```python
from build123d import *

# Parameters (mm, degrees)
SKETCH1_W           = 85
SKETCH1_H           = 60
BOSS_EXTRUDE1_DEPTH = 7.5
SKETCH2_R           = 2.25
CUT_EXTRUDE1_DEPTH  = 55.141019569
SKETCH3_W           = 85
SKETCH3_H           = 112
BOSS_EXTRUDE2_DEPTH = 10
FILLET1_R           = 10
SKETCH4_W           = 85
SKETCH4_H           = 65
BOSS_EXTRUDE3_DEPTH = 4.27
SKETCH5_W           = 85
SKETCH5_H           = 112
BOSS_EXTRUDE4_DEPTH = 14.27
FILLET2_R           = 10
FILLET3_R           = 2.5
FILLET4_R           = 2.5
FILLET5_R           = 2.5
SKETCH8_R           = 2.9
CUT_EXTRUDE2_DEPTH  = 25
SKETCH9_R           = 2.1
CUT_EXTRUDE3_DEPTH  = 14.27
SKETCH6_R           = 2.9
CUT_EXTRUDE4_DEPTH  = 25


with BuildPart() as part:
    # Sketch1 → Boss-Extrude1 (new, symmetric)
    with BuildSketch(Plane(origin=(0, 0, 0), x_dir=(1, 0, 0), z_dir=(0, 1, 0))):
        Rectangle(SKETCH1_W, SKETCH1_H)
    extrude(amount=BOSS_EXTRUDE1_DEPTH, both=True)

    # Sketch2 → Cut-Extrude1 (cut, through all)
    with BuildSketch(Plane(origin=(0, 7.5, 0), x_dir=(1, 0, 0), z_dir=(0, 1, 0))):
        with Locations(Location((3.95, -20.73, 0), (0, 0, 270))):
            Circle(SKETCH2_R)
        with Locations(Location((3.95, 21.27, 0), (0, 0, 270))):
            Circle(SKETCH2_R)
        with Locations(Location((27.95, 21.27, 0), (0, 0, 270))):
            Circle(SKETCH2_R)
        with Locations(Location((27.95, -20.73, 0), (0, 0, 270))):
            Circle(SKETCH2_R)
    extrude(amount=-CUT_EXTRUDE1_DEPTH, mode=Mode.SUBTRACT)

    # Sketch3 → Boss-Extrude2 (add)
    with BuildSketch(Plane.XY.offset(30)):
        with Locations((0, 48.5)):
            Rectangle(SKETCH3_W, SKETCH3_H)
    extrude(amount=BOSS_EXTRUDE2_DEPTH)

    # Fillet1
    fillet1_edges = [part.edges().sort_by_distance(p)[0] for p in [
        (0, -7.5, 40),
    ]]
    fillet(fillet1_edges, radius=FILLET1_R)

    # Sketch4 → Boss-Extrude3 (add)
    with BuildSketch(Plane(origin=(0, 0, 30), x_dir=(-1, 0, 0), z_dir=(0, 0, -1))):
        with Locations((0, 72)):
            Rectangle(SKETCH4_W, SKETCH4_H)
    extrude(amount=BOSS_EXTRUDE3_DEPTH)

    # Sketch5 → Boss-Extrude4 (add)
    with BuildSketch(Plane(origin=(0, 0, -30), x_dir=(-1, 0, 0), z_dir=(0, 0, -1))):
        with Locations((0, 48.5)):
            Rectangle(SKETCH5_W, SKETCH5_H)
    extrude(amount=BOSS_EXTRUDE4_DEPTH)

    # Fillet2
    fillet2_edges = [part.edges().sort_by_distance(p)[0] for p in [
        (0, -7.5, -44.27),
    ]]
    fillet(fillet2_edges, radius=FILLET2_R)

    # Fillet3
    fillet3_edges = [part.edges().sort_by_distance(p)[0] for p in [
        (0, 7.5, -30),
    ]]
    fillet(fillet3_edges, radius=FILLET3_R)

    # Fillet4
    fillet4_edges = [part.edges().sort_by_distance(p)[0] for p in [
        (0, 7.5, 30),
    ]]
    fillet(fillet4_edges, radius=FILLET4_R)

    # Fillet5
    fillet5_edges = [part.edges().sort_by_distance(p)[0] for p in [
        (0, 39.5, 30),
    ]]
    fillet(fillet5_edges, radius=FILLET5_R)

    # Sketch8 → Cut-Extrude2 (cut)
    with BuildSketch(Plane(origin=(0, 104.5, 0), x_dir=(1, 0, 0), z_dir=(0, 1, 0))):
        with Locations(Location((32.5, 37.135, 0), (0, 0, 270))):
            Circle(SKETCH8_R)
        with Locations(Location((-32.5, -32.865, 0), (0, 0, 270))):
            Circle(SKETCH8_R)
        with Locations(Location((-32.5, 37.135, 0), (0, 0, 270))):
            Circle(SKETCH8_R)
        with Locations(Location((16.5, -32.865, 0), (0, 0, 270))):
            Circle(SKETCH8_R)
    extrude(amount=-CUT_EXTRUDE2_DEPTH, mode=Mode.SUBTRACT)

    # Sketch9 → Cut-Extrude3 (cut)
    with BuildSketch(Plane.XY.offset(40)):
        with Locations((30.5, 88.06)):
            Circle(SKETCH9_R)
        with Locations((30.5, 65.06)):
            Circle(SKETCH9_R)
        with Locations((2.5, 65.06)):
            Circle(SKETCH9_R)
        with Locations((2.5, 88.06)):
            Circle(SKETCH9_R)
    extrude(amount=-CUT_EXTRUDE3_DEPTH, mode=Mode.SUBTRACT)

    # Sketch6 → Cut-Extrude4 (cut)
    with BuildSketch(Plane.ZY.offset(42.5)):
        with Locations((-37.135, 58.5)):
            Circle(SKETCH6_R)
        with Locations((32.865, 58.5)):
            Circle(SKETCH6_R)
        with Locations((-2.135, 0)):
            Circle(SKETCH6_R)
    extrude(amount=-CUT_EXTRUDE4_DEPTH, mode=Mode.SUBTRACT)


solid = part.part
```
Could you check a few things on this model? Use its own coordinates, in mm. A direction names the side the tool comes from. Give positions to 0.01 mm unless a question says otherwise; leave off trailing zeros. Loops run counter-clockwise (first coordinate to the right, second up) from the corner with the lowest first, then second, coordinate; pieces in that order, holes last. Notation, with made-up numbers: (3.25, 47.25) - (34.25, 47.25) arc R10 cw to (34.25, 53.25) - close; hole circle Ø7 at (-32, 47.25). An arc over 180 degrees is marked (long way). Answer in a Markdown table with one row per item. Add a question column.
Q1. For pin 1 (6 mm diameter, centred on x = 27.95, z = -21.27, fed in from +Y); pin 2 (2.5 mm diameter, centred on x = 3.95, z = -21.27, fed in from -Y); pin 3 (1.7 mm diameter, centred on x = -33.5, z = 34, fed in from +Y); pin 4 (3.5 mm diameter, centred on y = 0, z = -2.135, fed in from -X), each with a flat end and sliding along its axis, tell me the tip position at first contact or that it passes through.
Q2. If we section it at D-D (x = -11.5): List the corners of the cut face in (y, z) for me, plus the area to 3 significant figures.
Q3. Which directions (+Z, -Z, +X, -X, +Y, -Y) give clear straight access to the entire face, cutting with the end or side of a thin tool? Please do faces 1 (the face through (15.389, 92.175, 35.544)), 2 (the face through (-30.175, 55.927, -35.797)), 3 (the face through (-1, 39, 29)).
Q4. We'd pull the mould along Y, two halves only. Please class faces 4 (the face through (25.954, 0.105, -20.232)), 5 (the face through (-30.175, 55.927, 34.203)), 6 (the face through (1, 8, -29)): +Y half, -Y half, draft (parallel to the pull), parting line (faces both ways), or undercut.
Q5. If we section it at A-A (y = 47): List the corners of the cut face in (x, z) for me.
Q6. Please list where these lines run through material, in increasing order: L1, parallel to X at y = 2, z = -21; L2, parallel to Z at x = 36, y = 58; L3, parallel to Z at x = -14, y = 35. Write a range as from..to.
Q7. If we section it at B-B (z = -21.27): List the corners of the cut face in (x, y) for me, plus the area to 3 significant figures.
Q8. If we section it at C-C (x = -37): List the corners of the cut face in (y, z) for me (3 decimals), plus the area to 3 significant figures.
The answers:
| question | item | result |
|---|---|---|
| 1 | pin 1 | stops at y = 7.5 |
| 1 | pin 2 | passes through |
| 1 | pin 3 | stops at y = 79.5 |
| 1 | pin 4 | stops at x = -17.5 |
| 2 | outline | (-7.5, -34.27) arc R10 ccw to (2.5, -44.27) - (104.5, -44.27) - (104.5, -30) - (10, -30) arc R2.5 cw to (7.5, -27.5) - (7.5, 27.5) arc R2.5 cw to (10, 30) - (37, 30) arc R2.5 cw to (39.5, 27.5) - (39.5, 25.73) - (104.5, 25.73) - (104.5, 40) - (2.5, 40) arc R10 ccw to (-7.5, 30) - close |
| 2 | area | 3,860 mm^2 |
| 3 | face 1 | +Y |
| 3 | face 2 | -X |
| 3 | face 3 | +X, -X |
| 4 | face 4 | draft |
| 4 | face 5 | undercut |
| 4 | face 6 | +Y half |
| 5 | outline | (-42.5, -44.27) - (42.5, -44.27) - (42.5, -30) - (-42.5, -30) - close; (-42.5, 25.73) - (42.5, 25.73) - (42.5, 40) - (-42.5, 40) - close |
| 6 | L1 | x = -42.5..1.72, 6.18..25.72, 30.18..42.5 |
| 6 | L2 | z = -44.27..-30, 25.73..40 |
| 6 | L3 | z = -44.27..-30, 30..40 |
| 7 | outline | (-42.5, -7.5) - (1.7, -7.5) - (1.7, 7.5) - (-42.5, 7.5) - close; (6.2, -7.5) - (25.7, -7.5) - (25.7, 7.5) - (6.2, 7.5) - close; (30.2, -7.5) - (42.5, -7.5) - (42.5, 7.5) - (30.2, 7.5) - close |
| 7 | area | 1,140 mm^2 |
| 8 | outline | (-7.5, -34.27) arc R10 ccw to (2.5, -44.27) - (104.5, -44.27) - (104.5, -30) - (10, -30) arc R2.5 cw to (7.5, -27.5) - (7.5, 27.5) arc R2.5 cw to (10, 30) - (37, 30) arc R2.5 cw to (39.5, 27.5) - (39.5, 25.73) - (104.5, 25.73) - (104.5, 40) - (2.5, 40) arc R10 ccw to (-7.5, 30) - close; hole circle Ø5.8 at (0, -2.135); hole circle Ø5.8 at (58.5, -37.135); hole circle Ø5.8 at (58.5, 32.865) |
| 8 | area | 3,780 mm^2 |
